Source: three-view drawing plus pictorial views. Frame: mm from the lowest corner of the part. Give positions to 0.01 mm unless a question says otherwise; leave off trailing zeros. Order: outer loops, then holes, each group sorted by start corner. A loop starts at its lowest first (then second) coordinate and runs counter-clockwise, first axis right, second up. Notation, with made-up numbers: (31, -19.5) -> (65, -19.5) arc R9 cw to (65, -2.5) -> close; hole circle Ø2 at (-13.75, -31). An arc over 180 degrees is marked (long way). Write item = value, one per line.
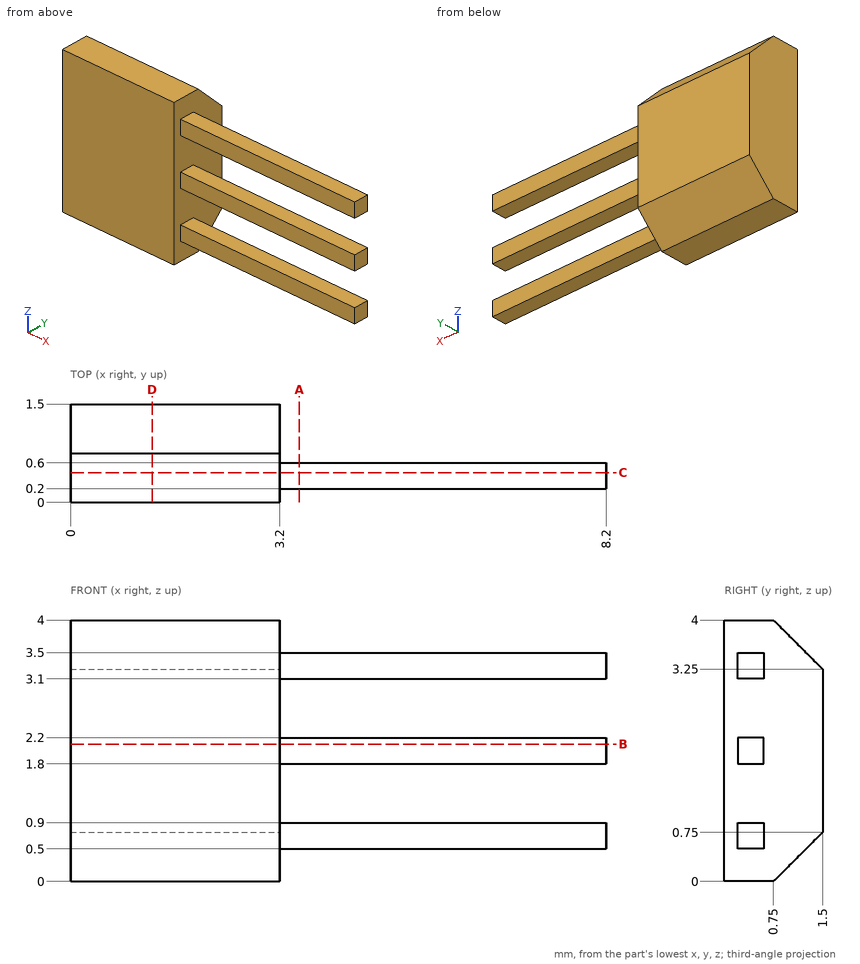
1) Section query B-B (z = 2.1). Output: boundary loops of the cut face in (x, y), plus the area to 3 significant figures.
Check sheet entries:
outline = (0, 0) -> (3.2, 0) -> (3.2, 0.2) -> (8.2, 0.2) -> (8.2, 0.6) -> (3.2, 0.6) -> (3.2, 1.5) -> (0, 1.5) -> close
area = 6.80 mm²
2) Section query D-D (x = 1.25). Output: boundary loops of the cut face in (y, z).
Check sheet entries:
outline = (0, 0) -> (0.75, 0) -> (1.5, 0.75) -> (1.5, 3.25) -> (0.75, 4) -> (0, 4) -> close
3) Section query A-A (x = 3.5). Output: boundary loops of the cut face in (y, z), plus the area to 3 significant figures.
Check sheet entries:
outline = (0.2, 0.5) -> (0.6, 0.5) -> (0.6, 0.9) -> (0.2, 0.9) -> close; (0.2, 1.8) -> (0.6, 1.8) -> (0.6, 2.2) -> (0.2, 2.2) -> close; (0.2, 3.1) -> (0.6, 3.1) -> (0.6, 3.5) -> (0.2, 3.5) -> close
area = 0.480 mm²
4) Section query C-C (y = 0.45). Output: boundary loops of the cut face in (x, z), plus the area to 3 significant figures.
Check sheet entries:
outline = (0, 0) -> (3.2, 0) -> (3.2, 0.5) -> (8.2, 0.5) -> (8.2, 0.9) -> (3.2, 0.9) -> (3.2, 1.8) -> (8.2, 1.8) -> (8.2, 2.2) -> (3.2, 2.2) -> (3.2, 3.1) -> (8.2, 3.1) -> (8.2, 3.5) -> (3.2, 3.5) -> (3.2, 4) -> (0, 4) -> close
area = 18.8 mm²
5) First-contact query: P1, Ø1, axis at x = 7, z = 3, coming from the +Y side. Flat tip, straight axial feed; report the tip coordinate or a pass-through.
Check sheet entries:
P1 = 0.6
6) Line query: line 1 (Z direction, x = 4, y = 0.25); line 2 (X direction, y = 0.75, z = 3.25); line 3 (Z direction, x = 2.25, y = 0.95). Output: solid intervals per line, ascending. Write a range as from..to.
Check sheet entries:
line_1 = 0.5..0.9, 1.8..2.2, 3.1..3.5
line_2 = 0..3.2
line_3 = 0.2..3.8
